Autodesk Fusion 360 part; units mm, degrees
sketch "Sketch1" plane through (0, 0, 0) normal (0, 0, 1) x (1, 0, 0)
  line L0 (100, 125) -> (-100, 125)
  line L1 (-100, 125) -> (-100, -125)
  line L2 (-100, -125) -> (100, -125)
  line L3 (100, -125) -> (100, 125)
  line L4 (100, 125) -> (-100, -125) construction
  line L5 (-100, 125) -> (100, -125) construction
  line L6 (-100, 125) -> (100, 125)
  line L7 (100, 125) -> (100, 129)
  line L8 (100, 129) -> (-100, 129)
  line L9 (-100, 129) -> (-100, 125)
  line L10 (-100, -125) -> (100, -125)
  line L11 (100, -125) -> (100, -129)
  line L12 (100, -129) -> (-100, -129)
  line L13 (-100, -129) -> (-100, -125)
  line L14 (100, 125) -> (104, 125)
  line L15 (104, 125) -> (104, -125)
  line L16 (104, -125) -> (100, -125)
  line L17 (100, -125) -> (100, 125)
  line L18 (-100, 125) -> (-104, 125)
  line L19 (-104, 125) -> (-104, -125)
  line L20 (-104, -125) -> (-100, -125)
  line L21 (-100, -125) -> (-100, 125)
  line L22 (-80, -53.8) -> (-80, 2.2) construction
  circle A0 centre (-80, -53.8) radius 1.65 construction
  circle A1 centre (-80, 2.2) radius 1.65 construction
  line L23 (-61.0622, -1) -> (-98.9378, -1) construction
  line L24 (-98.9378, -1) -> (-98.9378, -50.6) construction
  line L25 (-98.9378, -50.6) -> (-61.0622, -50.6) construction
  line L26 (-61.0622, -50.6) -> (-61.0622, -1) construction
  line L27 (-61.0622, -1) -> (-98.9378, -50.6) construction
  line L28 (-98.9378, -1) -> (-61.0622, -50.6) construction
  line L29 (-30.5, 49.5) -> (98.5, 49.5) construction
  line L30 (98.5, 49.5) -> (98.5, -47.5) construction
  line L31 (98.5, -47.5) -> (-30.5, -47.5) construction
  line L32 (-30.5, -47.5) -> (-30.5, 49.5) construction
  circle A2 centre (-28, 43) radius 1.65
  circle A3 centre (94, -42) radius 1.65
  line L33 (-100, 125) -> (-85.5, 125)
  line L34 (-85.5, 125) -> (-85.5, 116)
  line L35 (-85.5, 116) -> (-100, 116)
  line L36 (-100, 116) -> (-100, 125)
  line L37 (100, 125) -> (85.5, 125)
  line L38 (85.5, 125) -> (85.5, 116)
  line L39 (85.5, 116) -> (100, 116)
  line L40 (100, 116) -> (100, 125)
  line L41 (-100, -125) -> (-85.5, -125)
  line L42 (-85.5, -125) -> (-85.5, -116)
  line L43 (-85.5, -116) -> (-100, -116)
  line L44 (-100, -116) -> (-100, -125)
  line L45 (100, -125) -> (85.5, -125)
  line L46 (85.5, -125) -> (85.5, -116)
  line L47 (85.5, -116) -> (100, -116)
  line L48 (100, -116) -> (100, -125)
  line L49 (-100, 100) -> (-104, 100)
  line L50 (100, 100) -> (104, 100)
  line L51 (-100, -100) -> (-104, -100)
  line L52 (100, -100) -> (104, -100)
  line L53 (-85.5, 125) -> (-85.5, 129)
  line L54 (85.5, 125) -> (85.5, 129)
  line L55 (-85.5, -125) -> (-85.5, -129)
  line L56 (85.5, -125) -> (85.5, -129)
  line L57 (-115, -140) -> (-75, -140) construction
  line L58 (-75, -140) -> (-75, -87) construction
  line L59 (-75, -87) -> (-115, -87) construction
  line L60 (-115, -87) -> (-115, -140) construction
  line L61 (-63.3606, -140) -> (-21.3606, -140) construction
  line L62 (-21.3606, -140) -> (-21.3606, -53.8) construction
  line L63 (-21.3606, -53.8) -> (-63.3606, -53.8) construction
  line L64 (-63.3606, -53.8) -> (-63.3606, -140) construction
  line L65 (-100, 0) -> (-118.2487, 0) construction
  circle A4 centre (0, 0) radius 152.5
  circle A5 centre (-85, -72) radius 1.65
  line L66 (-85, -72) -> (85, -72) construction
  line L67 (85, -72) -> (85, 72) construction
  line L68 (85, 72) -> (-85, 72) construction
  line L69 (-85, 72) -> (-85, -72) construction
  circle A6 centre (85, 72) radius 1.65
  circle A7 centre (85, -72) radius 1.65
  circle A8 centre (-85, 72) radius 1.65
  point P0 (-80, -25.8)
  dimension "d1" = 200
  dimension "d2" = 250
  dimension "d3" = 4
  dimension "d4" = 4
  dimension "d5" = 4
  dimension "d6" = 4
  dimension "d7" = 20
  dimension "d8" = 56
  dimension "d10" = 3.3
  dimension "d11" = 37.8755
  dimension "d12" = 49.6
  dimension "d13" = 2.5
  dimension "d14" = 6.5
  dimension "d15" = 3.3
  dimension "d16" = 5.5
  dimension "d17" = 4.5
  dimension "d18" = 129
  dimension "d19" = 97
  dimension "d20" = 1.5
  dimension "d21" = 14.5
  dimension "d22" = 9
  dimension "d23" = 14.5
  dimension "d24" = 9
  dimension "d25" = 14.5
  dimension "d26" = 14.5
  dimension "d27" = 9
  dimension "d28" = 9
  dimension "d29" = 25
  dimension "d30" = 25
  dimension "d31" = 25
  dimension "d32" = 25
  dimension "d33" = 40
  dimension "d34" = 53
  dimension "d35" = 15
  dimension "d36" = 15
  dimension "d37" = 3.3
  dimension "d38" = 86.2
  dimension "d39" = 42
  dimension "d40" = 1
  dimension "d50" = 305
  dimension "d51" = 3.3
  dimension "d52" = 15
  dimension "d53" = 15
  dimension "d54" = 15
  dimension "d55" = 53
  dimension "d56" = 53
  dimension "d57" = 170
  dimension "d58" = 144
  dimension "d60" = 47.5
  dimension "d61" = 49.5
extrude "Extrude1" add sketch "Sketch1" along normal blind 3 contours L0 L1 L2 L3 L6 L10 L17 L21 L34 L35 L38 L39 L42 L43 L46 L47 A4 | L0 L6 L8 L53 L54 A4 | L3 L15 L17 L50 L52 | L1 L19 L21 L49 L51 | L2 L10 L12 L55 L56 A4
hole "Hole1" at (0, 129, 0) direction (0, 0, 1) diameter 30 depth 10 tip angle 118
hole "Hole2" at (0.013, 55.0023, 0) direction (0, 0, 1) diameter 12 depth 10 tip angle 118
fillet "Fillet1" [suppressed]
fillet "Fillet2" [suppressed]
chamfer "Chamfer1" [suppressed]
fillet "Fillet3" [suppressed]
equation "d4 = d3"
equation "d5 = d3"
equation "d6 = d3"
equation "d23 = d21"
equation "d24 = d22"
equation "d25 = d21"
equation "d26 = d25"
equation "d27 = d22"
equation "d28 = d24"
equation "d30 = d29"
equation "d31 = d29"
equation "d32 = d29"
equation "d36 = d35"
equation "d60 = d19 / 2 - 1 mm"
Check sheet for the modelled part. Datum: model origin and axes. Units: mm. Round coordinates to 2 decimals unless told otherwise and drop trailing zeros. Loops run counter-clockwise (first coordinate to the right, second up) from the corner with the lowest first, then second, coordinate; pieces in that order, holes last. Notation, with made-up numbers: (8, 23) - (21, 23) arc R20 ccw to (21, 58) - close; hole circle Ø10 at (65, 34.5). An arc over 180 degrees is marked (long way). Answer as a JSON object with one key per item and string values. Group by question number.
Q1. Sectioned sample at B-B, the plane z = 0.7. Count the separate pieces of the cut face and the enclosed holes in it, plus the area to 3 significant figures.
Q2. Sectioned sample at A-A, the plane x = 89.5. Enter the section's corners in (y, z), plus the area to 3 significant figures.
Q3. Scan lines: line 1 along X through (y, z) = (-72, 2.2); line 2 along Y through (x, z) = (-85, 2.15); line 3 along X through (y, z) = (-70.5, 2.6). Record each from-to range of solid material in increasing order. Write a range as [from, to].
Q4. Gauge pin test, flat ends, axial feed: P1, Ø2.5, axis at x = -85, y = -72, coming from the -Z side; P2, Ø1.5, axis at x = -102, z = 1, coming from the -Y side; P3, Ø0.9, axis at x = -95.5, z = 2, coming from the -Y side; P4, Ø1.5, axis at y = -105, z = 2, coming from the -X side. Record the tip position at first contact, or that the pin passes through.
Q5. Mould release check, pull along Y, two halves, no side actions. Record for faces 1 (the face through (-0.25, 49.01, 1.52)), 2 (the face through (-1, 2, 0)), 3 (the face through (0, 114, 2)): released by +Y, released by -Y, zero draft, split by the parting line, or undercut.
Q6. Sectioned sample at C-C, the plane x = -12. Enter the section's corners in (y, z).
Solution:
{
 "1": {"separate pieces": "1", "enclosed holes": "7", "area": "51,900 mm²"},
 "2": {"outline": "(-116, 0) - (116, 0) - (116, 3) - (-116, 3) - close", "area": "696 mm²"},
 "3": {"line 1": "x = [-104, -86.65], [-83.35, 83.35], [86.65, 104]", "line 2": "y = [-126.61, -73.65], [-70.35, 70.35], [73.65, 126.61]", "line 3": "x = [-104, -85.69], [-84.31, 84.31], [85.69, 104]"},
 "4": {"P1": "passes through", "P2": "stops at y = -100", "P3": "stops at y = -116", "P4": "stops at x = -100"},
 "5": {"face 1": "undercut", "face 2": "zero draft", "face 3": "released by +Y"},
 "6": {"outline": "(-129, 0) - (120, 0) - (120, 3) - (-129, 3) - close"}
}
